Geometry check sheet. Reference: the model listing, model coordinates, mm. Give positions to 0.01 mm unless a question says otherwise; leave off trailing zeros. Write each loop counter-clockwise with the first axis right and the second up, starting at its lowest first coordinate (ties: lowest second). Pieces come first, ordered by that corner, then holes. Notation, with made-up numbers: (58, -4.75) - (77, -4.75) arc R6 ccw to (77, -0.75) - close; hole circle Ø2 at (68.5, 83). An arc over 180 degrees is marked (long way). One line per question, with ' | ' between items. Start each with the question number.
Q1. Gauge pin test, flat ends, axial feed: P1, Ø4, axis at x = 11, y = 4, coming from the +Z side; P2, Ø1.6, axis at y = 1, z = -4, coming from the -X side; P3, Ø0.7, axis at x = -6.5, z = -2, coming from the +Y side. Record the tip position at first contact, or that the pin passes through.
Q2. Section check A-A on y = 2.5. Record the boundary of the cut face in (x, z).
Q3. Section check B-B on z = -1.5. Record the boundary of the cut face in (x, y).
Q4. Section check C-C on x = -7.5. Record the boundary of the cut face in (y, z).
Q5. Thickness scan on L1, parallel to Y at x = 4.5, z = 2.75; L2, parallel to X at y = 7.75, z = -2; L3, parallel to X at y = 0.75, z = -6. Record the ranges inside material, lowest first. Write a range as [from, to].
Q6. Section check D-D on z = -5.75. Record the boundary of the cut face in (x, y).
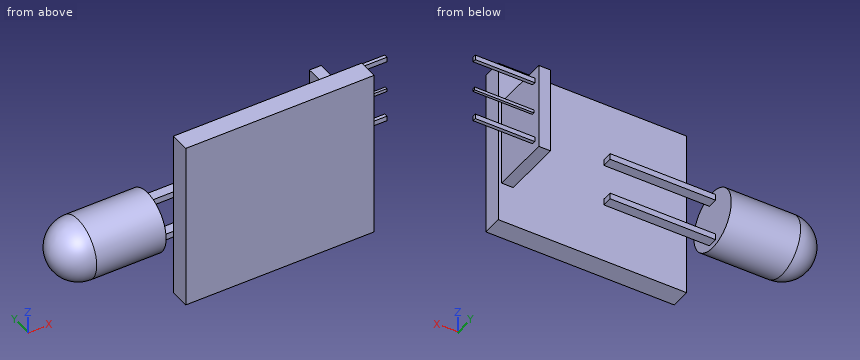
```python
from build123d import *

# Parameters (mm, degrees)
ESQUISSE1_W        = 19
ESQUISSE1_H        = 17
BOSS_EXTRU_1_DEPTH = 2
ESQUISSE2_W        = 1.17663859
ESQUISSE2_H        = 8.785143252
BOSS_EXTRU_2_DEPTH = 6
ESQUISSE3_W        = 0.492340061
ESQUISSE3_H        = 0.351671472
BOSS_EXTRU_3_DEPTH = 6
ESQUISSE4_W        = 0.313154041
ESQUISSE4_H        = 0.257723979
BOSS_EXTRU_4_DEPTH = 6
ESQUISSE5_W        = 0.663647826
ESQUISSE5_H        = 0.612597993
BOSS_EXTRU_5_DEPTH = 1
ESQUISSE6_W        = 0.612597993
ESQUISSE6_H        = 1
BOSS_EXTRU_6_DEPTH = 10
ESQUISSE7_R        = 3
BOSS_EXTRU_7_DEPTH = 10
CONG_2_R           = 3


with BuildPart() as part:
    # Esquisse1 → Boss.-Extru.1 (new body)
    with BuildSketch(Plane(origin=(0, 0, 0), x_dir=(1, 0, 0), z_dir=(0, 1, 0))):
        Rectangle(ESQUISSE1_W, ESQUISSE1_H)
    extrude(amount=BOSS_EXTRU_1_DEPTH)

    # Esquisse2 → Boss.-Extru.2 (add)
    with BuildSketch(Plane(origin=(0, 2, 0), x_dir=(1, 0, 0), z_dir=(0, 1, 0))):
        with Locations((8.589461706, 0)):
            Rectangle(ESQUISSE2_W, ESQUISSE2_H)
    extrude(amount=BOSS_EXTRU_2_DEPTH)

    # Esquisse3 → Boss.-Extru.3 (add)
    with BuildSketch(Plane(origin=(9.177781001, 0, 0), x_dir=(0, 0, -1), z_dir=(1, 0, 0))):
        with Locations((-3.200210394, 7.175487816)):
            Rectangle(ESQUISSE3_W, ESQUISSE3_H)
    boss_extru_3 = extrude(amount=BOSS_EXTRU_3_DEPTH)

    # Symétrie1: Boss.-Extru.3 across plane
    add(boss_extru_3.mirror(Plane.XY))

    # Esquisse4 → Boss.-Extru.4 (add)
    with BuildSketch(Plane(origin=(9.177781001, 0, 0), x_dir=(0, 0, -1), z_dir=(1, 0, 0))):
        with Locations((0.092212431, 7.099938204)):
            Rectangle(ESQUISSE4_W, ESQUISSE4_H)
    extrude(amount=BOSS_EXTRU_4_DEPTH)

    # Esquisse5 → Boss.-Extru.5 (add)
    with BuildSketch(Plane(origin=(0, 2, 0), x_dir=(1, 0, 0), z_dir=(0, 1, 0))):
        with Locations((-1.474820367, -2.144092976)):
            Rectangle(ESQUISSE5_W, ESQUISSE5_H)
    boss_extru_5 = extrude(amount=BOSS_EXTRU_5_DEPTH)

    # Esquisse6 → Boss.-Extru.6 (add)
    with BuildSketch(Plane.ZY.offset(1.80664428)):
        with Locations((2.144092976, 2.5)):
            Rectangle(ESQUISSE6_W, ESQUISSE6_H)
    boss_extru_6 = extrude(amount=BOSS_EXTRU_6_DEPTH)

    # Symétrie2: Boss.-Extru.5, Boss.-Extru.6 across plane
    add(boss_extru_5.mirror(Plane.XY))
    add(boss_extru_6.mirror(Plane.XY))

    # Esquisse7 → Boss.-Extru.7 (add)
    with BuildSketch(Plane.ZY.offset(11.80664428)):
        with Locations((0, 2.5)):
            Circle(ESQUISSE7_R)
    extrude(amount=BOSS_EXTRU_7_DEPTH)

    # Congé2
    cong_2_edges = [part.edges().sort_by_distance(p)[0] for p in [
        (-21.80664428, 2.5, -3),
    ]]
    fillet(cong_2_edges, radius=CONG_2_R)


solid = part.part
```
Working result:
1) P1: stops at z = 4.39 | P2: stops at x = -9.5 | P3: stops at y = 3
2) outline: (-18.81, -3) - (-11.81, -3) - (-11.81, -2.45) - (-1.14, -2.45) - (-1.14, -1.84) - (-11.81, -1.84) - (-11.81, 1.84) - (-1.14, 1.84) - (-1.14, 2.45) - (-11.81, 2.45) - (-11.81, 3) - (-18.81, 3) arc R3 ccw to start; (8, -4.39) - (9.18, -4.39) - (9.18, 4.39) - (8, 4.39) - close
3) outline: (-18.81, -0.1) - (-11.81, -0.1) - (-11.81, 5.1) - (-18.81, 5.1) arc R2.6 ccw to start; (-9.5, 0) - (9.5, 0) - (9.5, 2) - (9.18, 2) - (9.18, 8) - (8, 8) - (8, 2) - (-9.5, 2) - close
4) outline: (0, -8.5) - (2, -8.5) - (2, -2.45) - (3, -2.45) - (3, -1.84) - (2, -1.84) - (2, 1.84) - (3, 1.84) - (3, 2.45) - (2, 2.45) - (2, 8.5) - (0, 8.5) - close
5) L1: y = [0, 2] | L2: x = [8, 9.18] | L3: x = [-9.5, 9.5]
6) outline: (-9.5, 0) - (9.5, 0) - (9.5, 2) - (-9.5, 2) - close
